Geometry check sheet. Reference: drawing and pictorial views, mm from the part's lowest x, y, z. A direction names the side the tool comes from. Give positions to 0.01 mm unless a question says otherwise; leave off trailing zeros. Order: outer loops, then holes, each group sorted by start corner. A loop starts at its lowest first (then second) coordinate and runs counter-clockwise, first axis right, second up. Notation, with made-up numbers: M 60.5,-34.5 L 80.5,-34.5 A30 ccw 80.5,-2.5 Z; hole C 40,32.5 d4. An arc over 180 degrees is marked long. Answer as CSV lines item,"result".
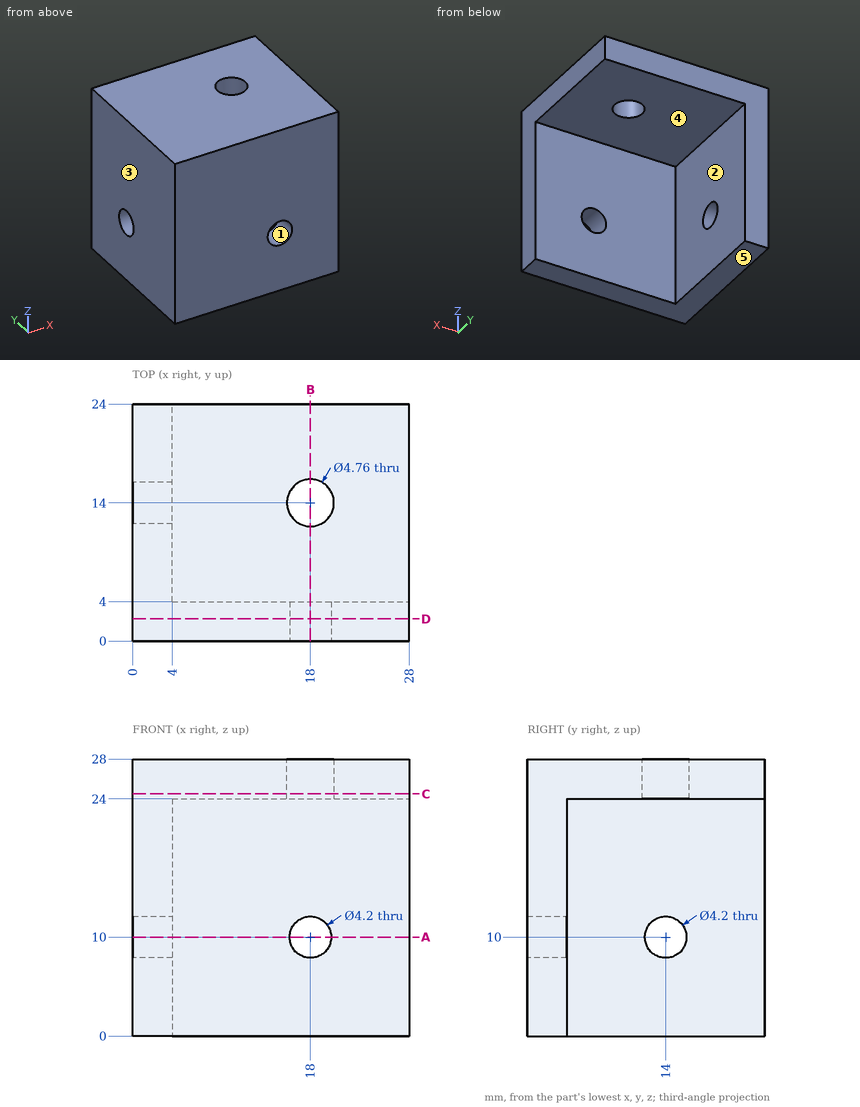
(1) Tool access check on the marked faces 4 and 5. Record the directions out of +Z, -Z, +X, -X, +Y, -Y that give a thin tool (end or side, any length) a straight path to the whole face; none if there is none.
The answers:
face 4,"-Z, +X, +Y"
face 5,"-Z, +X, -X, +Y, -Y"
(2) Section check C-C on z = 24.5. Enter the section's corners in (x, y).
The answers:
outline,"M 0,0 L 28,0 L 28,24 L 0,24 Z; hole C 18,14 d4.76"
(3) Gauge pin test, flat ends, axial feed: P1, Ø7, axis at x = 14.5, z = 11, coming from the +Y side; P2, Ø3.5, axis at y = 14, z = 10, coming from the +X side (3 decimals); P3, Ø2, axis at x = 10.5, y = 15.5, coming from the -Z side. Record the tip position at first contact, or that the pin passes through.
The answers:
P1,"stops at y = 4"
P2,"passes through"
P3,"stops at z = 24"
(4) Material ranges on line 1 (X direction, y = 2.25, z = 10); line 2 (Y direction, x = 15.5, z = 16.5); line 3 (Z direction, x = 10.25, y = 4.5), recorded low to high.
The answers:
line 1,"x = 0 to 15.9, 20.1 to 28"
line 2,"y = 0 to 4"
line 3,"z = 24 to 28"
(5) Section check A-A on z = 10. Enter the section's corners in (x, y).
The answers:
outline,"M 0,0 L 15.9,0 L 15.9,4 L 4,4 L 4,11.9 L 0,11.9 Z; M 0,16.1 L 4,16.1 L 4,24 L 0,24 Z; M 20.1,0 L 28,0 L 28,4 L 20.1,4 Z"
(6) Section check B-B on x = 18. Enter the section's corners in (y, z).
The answers:
outline,"M 0,0 L 4,0 L 4,7.9 L 0,7.9 Z; M 0,12.1 L 4,12.1 L 4,24 L 11.62,24 L 11.62,28 L 0,28 Z; M 16.38,24 L 24,24 L 24,28 L 16.38,28 Z"
(7) Draft check along X on the marked faces 1, 2 and 3. Enter one of: +X half, -X half, draft (parallel to the pull), parting line (faces both ways), or undercut.
The answers:
face 1,"undercut"
face 2,"+X half"
face 3,"-X half"
(8) Section check D-D on y = 2.25. Enter the section's corners in (x, z).
The answers:
outline,"M 0,0 L 28,0 L 28,28 L 0,28 Z; hole C 18,10 d4.2"
